```python
from build123d import *

# Parameters (mm, degrees)
BOSS_EXTRUDE1_DEPTH = 5
BOSS_EXTRUDE2_DEPTH = 5
CUT_EXTRUDE1_REACH  = 7
SKETCH3_R           = 2


with BuildPart() as part:
    # Sketch1 → Boss-Extrude1 (new body)
    with BuildSketch(Plane.XY):
        with BuildLine():
            Line((-2.520114714, 12.117440709), (-2.520114714, 6.269831909))
            Line((-2.520114714, 6.269831909), (-0.666012747, 0.563492811))
            ThreePointArc((-0.666012747, 0.563492811), (-6.290753591, 1.602682623), (-8.48865141, 6.883484665))
            Line((-8.48865141, 6.883484665), (-6.437898745, 12.117778688))
            Line((-6.437898745, 12.117778688), (-6.520114714, 22.117440709))
            ThreePointArc((-6.520114714, 22.117440709), (-6.459345726, 22.81203342), (-6.278885197, 23.485521282))
            Line((-6.278885197, 23.485521282), (-3.883018647, 30.068110528))
            Line((-3.883018647, 30.068110528), (-10.954086459, 37.13917834))
            ThreePointArc((-10.954086459, 37.13917834), (-12.015892078, 39.702603869), (-10.954086459, 42.266029397))
            Line((-10.954086459, 42.266029397), (-0.347484741, 52.872631115))
            ThreePointArc((-0.347484741, 52.872631115), (3.603256686, 53.658482445), (5.841171936, 50.309205586))
            Line((5.841171936, 50.309205586), (5.841171936, 45.309205586))
            Line((5.841171936, 45.309205586), (2.215940787, 45.309205586))
            Line((2.215940787, 45.309205586), (2.215940787, 50.309205586))
            Line((2.215940787, 50.309205586), (-8.39066093, 39.702603869))
            Line((-8.39066093, 39.702603869), (-0.124248164, 31.436191102))
            ThreePointArc((-0.124248164, 31.436191102), (0.116981353, 30.068110528), (-0.124248164, 28.700029955))
            Line((-0.124248164, 28.700029955), (-2.520114714, 22.117440709))
            Line((-2.520114714, 22.117440709), (-2.520114714, 12.117440709))
        make_face()
    extrude(amount=BOSS_EXTRUDE1_DEPTH)

    # Sketch2 → Boss-Extrude2 (add)
    with BuildSketch(Plane.XY.offset(5)):
        with BuildLine():
            Line((-0.666012747, 0.563492811), (-0.444155406, 0.640409829))
            ThreePointArc((-0.444155406, 0.640409829), (-0.320137366, 1.836179716), (-0.904060997, 2.887026655))
            ThreePointArc((-0.904060997, 2.887026655), (-0.316507803, 3.236827197), (0.197736204, 3.687529179))
            ThreePointArc((0.197736204, 3.687529179), (1.016708708, 2.807455242), (2.192277133, 2.55589019))
            Line((2.192277133, 2.55589019), (2.468262924, 2.935752043))
            ThreePointArc((2.468262924, 2.935752043), (1.865739721, 3.976046178), (0.775663247, 4.482977511))
            ThreePointArc((0.775663247, 4.482977511), (1.045396166, 5.111327197), (1.196512329, 5.778217803))
            ThreePointArc((1.196512329, 5.778217803), (2.376369483, 5.547602991), (3.475290544, 6.035064372))
            Line((3.475290544, 6.035064372), (3.475290544, 6.504599445))
            ThreePointArc((3.475290544, 6.504599445), (2.376369483, 6.992060826), (1.196512329, 6.761446014))
            ThreePointArc((1.196512329, 6.761446014), (1.045396166, 7.428336621), (0.775663247, 8.056686306))
            ThreePointArc((0.775663247, 8.056686306), (1.865739721, 8.56361764), (2.468262924, 9.603911774))
            Line((2.468262924, 9.603911774), (2.192277133, 9.983773627))
            ThreePointArc((2.192277133, 9.983773627), (1.016708708, 9.732208576), (0.197736204, 8.852134639))
            ThreePointArc((0.197736204, 8.852134639), (-0.316507803, 9.302836621), (-0.904060997, 9.652637162))
            ThreePointArc((-0.904060997, 9.652637162), (-0.320137366, 10.703484102), (-0.444155406, 11.899253988))
            Line((-0.444155406, 11.899253988), (-0.890709796, 12.044348305))
            ThreePointArc((-0.890709796, 12.044348305), (-1.693898402, 11.14984612), (-1.839166595, 9.956471389))
            ThreePointArc((-1.839166595, 9.956471389), (-2.178215907, 10.003209228), (-2.520114714, 10.018831909))
            Line((-2.520114714, 10.018831909), (-2.520114714, 8.269831909))
            ThreePointArc((-2.520114714, 8.269831909), (-0.544738032, 6.582700839), (-1.902080725, 4.367718876))
            Line((-1.902080725, 4.367718876), (-0.666012747, 0.563492811))
        make_face()
    extrude(amount=-BOSS_EXTRUDE2_DEPTH)

    # Sketch3 → Cut-Extrude1 (cut, up to next)
    with BuildSketch(Plane.XY.offset(5), mode=Mode.PRIVATE) as cut_extrude1_sk1:
        with Locations((-2.520114714, 6.269831909)):
            Circle(SKETCH3_R)
    cut_extrude1_tool1 = extrude(cut_extrude1_sk1.sketch, amount=-CUT_EXTRUDE1_REACH, mode=Mode.PRIVATE) & part.part
    add(cut_extrude1_tool1.solids().sort_by_distance((-2.520115, 6.269832, 5))[0], mode=Mode.SUBTRACT)


solid = part.part
```
Input: part model. Units: mm. Frame: model coordinates. A direction names the side the tool comes from. Round coordinates to 2 decimals unless told otherwise and drop trailing zeros. Loops run counter-clockwise (first coordinate to the right, second up) from the corner with the lowest first, then second, coordinate; pieces in that order, holes last. Notation, with made-up numbers: (-24.5, 1.25) -> (23.5, 1.25) arc R20 ccw to (23.5, 30.25) -> close; hole circle Ø7 at (58.5, 53.5). An arc over 180 degrees is marked (long way). One line per item, written item: value.
(1) Mould query, pull axis Y, two halves, no side actions, for faces 1 (the face through (-5.725, 47.495, 2.465)), 2 (the face through (1.03, 9.74, 2.54)), 3 (the face through (-1.305, 25.455, 2.465)), 4 (the face through (-3, 27, 5)). Classes: pulls with the +Y half, pulls with the -Y half, needs draft (parallel to the pull), parting line crosses it, or undercut.
Geometry check:
face 1: pulls with the +Y half
face 2: undercut
face 3: undercut
face 4: needs draft
(2) Section C-C (y = 46). Return the cut outline in (x, z).
Geometry check:
outline: (-7.22, 0) -> (-2.09, 0) -> (-2.09, 5) -> (-7.22, 5) -> close; (2.22, 0) -> (5.84, 0) -> (5.84, 5) -> (2.22, 5) -> close
(3) Material intervals for line 1 (Y direction, x = 1.5, z = 2.7); line 2 (Y direction, x = -3, z = 2.55); line 3 (X direction, y = 13.5, z = 2.6), sorted ascending. Write a range as [from, to].
Geometry check:
line 1: [2.61, 4.24], [5.64, 6.9], [8.3, 9.93], [49.59, 53.86]
line 2: [0.29, 4.33], [8.21, 34.31], [45.09, 50.22]
line 3: [-6.45, -2.52]
(4) Section D-D (x = -9). Return the cut outline in (y, z).
Geometry check:
outline: (35.19, 0) -> (44.22, 0) -> (44.22, 5) -> (35.19, 5) -> close
(5) Section B-B (y = 10.5). Return the cut outline in (x, z).
Geometry check:
outline: (-7.07, 0) -> (-2.52, 0) -> (-2.52, 5) -> (-7.07, 5) -> close; (-1.87, 0) -> (-0.37, 0) -> (-0.37, 5) -> (-1.87, 5) -> close
(6) Section A-A (x = -3.25). Return the cut outline in (y, z), plus the area to 3 significant figures.
Geometry check:
outline: (0.31, 0) -> (4.41, 0) -> (4.41, 5) -> (0.31, 5) -> close; (8.13, 0) -> (34.56, 0) -> (34.56, 5) -> (8.13, 5) -> close; (44.84, 0) -> (49.97, 0) -> (49.97, 5) -> (44.84, 5) -> close
area: 178 mm2
(7) Set-up query: faces 5 (the face through (-4.32, 35.63, 2.46)), 6 (the face through (-3, 27, 0)), 7 (the face through (-6.46, 22.8, 2.46)). Return all of +Z, -Z, +X, -X, +Y, -Y with unobstructed straight access to the full face (end or side cutting, diameter ignored); none if empty.
Geometry check:
face 5: +Z, -Z, +X
face 6: -Z, +X, -X, +Y, -Y
face 7: +Z, -Z, -X
(8) Pin query (flat end, axial travel): pin 1 (3 mm diameter, centred on y = 41.5, z = 0.5, fed in from +X); pin 2 (1 mm diameter, centred on y = 41.5, z = 3, fed in from -X); pin 3 (2.5 mm diameter, centred on y = 18, z = 2, fed in from +X). Return the tip coordinate at first contact, or that it passes through.
Geometry check:
pin 1: x = -5.09
pin 2: x = -11.78
pin 3: x = -2.52
